Read the model definition and answer for the solid it produces. Units are mm, in the model's axes. A direction names the side the tool comes from. Coordinates: 2 decimals unless noted, no trailing zeros. Write each loop counter-clockwise with the first axis right and the second up, starting at its lowest first coordinate (ties: lowest second). Pieces come first, ordered by that corner, then holes. Notation, with made-up numbers: (87, 84) -> (98, 84) arc R29 cw to (98, 122) -> close; hole circle Ø1 at (72.5, 26). An arc over 180 degrees is marked (long way). Use CSV: the item, a comma, the result in double quotes.
from build123d import *

# Parameters (mm, degrees)
SKETCH1_W           = 4.572
SKETCH1_H           = 28.575
SKETCH2_R           = 12.1666
BOSS_EXTRUDE1_DEPTH = 20.828
CUT_EXTRUDE1_DEPTH  = 26.4
SKETCH4_W           = 25.4
SKETCH4_H           = 4.0005
HOLE1_D             = 5.1816
HOLE1_DEPTH         = 25.4


with BuildPart() as part:
    # Sketch1 → Revolve1 (revolve)
    with BuildSketch(Plane.XY):
        with Locations((-15.321066246, 14.2875)):
            Rectangle(SKETCH1_W, SKETCH1_H)
    revolve(axis=Axis((-17.607066246, 0, 0), (1, 0, 0)))

    # Sketch2 → Boss-Extrude1 (add)
    with BuildSketch(Plane(origin=(-13.035066246, 0, 0), x_dir=(0, 0, -1), z_dir=(1, 0, 0))):
        Circle(SKETCH2_R)
    extrude(amount=BOSS_EXTRUDE1_DEPTH)

    # Sketch3 → Cut-Extrude1 (cut, through all)
    with BuildSketch(Plane.ZY.offset(17.607066246)):
        with BuildLine():
            Line((1.0033, 3.872646299), (1.0033, 5.0038))
            Line((1.0033, 5.0038), (-1.0033, 5.0038))
            Line((-1.0033, 5.0038), (-1.0033, 3.872646299))
            ThreePointArc((-1.0033, 3.872646299), (0, 4.0005), (1.0033, 3.872646299))
        make_face()
    extrude(amount=-CUT_EXTRUDE1_DEPTH, mode=Mode.SUBTRACT)

    # Sketch4 → Cut-Revolve1 (revolve, cut)
    with BuildSketch(Plane(origin=(0, 0, 0), x_dir=(-1, 0, 0), z_dir=(0, 0, -1))):
        with Locations((4.907066246, 2.00025)):
            Rectangle(SKETCH4_W, SKETCH4_H)
    revolve(axis=Axis((7.792933754, 0, 0), (-1, 0, 0)), mode=Mode.SUBTRACT)

    # Hole1
    with Locations(Plane.ZY.offset(17.607066246)):
        with Locations((23.8125, 0), (11.90625, 20.622229928), (-11.90625, 20.622229928), (-23.8125, 0), (-11.90625, -20.622229928), (11.90625, -20.622229928)):
            Hole(HOLE1_D / 2, depth=HOLE1_DEPTH)


solid = part.part
1. A tool of negligible diameter and unlimited length cuts with its end or side. For faces 1 (the cylindrical face through (-3, 12, 2)), 2 (the flat face through (-17.607, 0, -6)), 3 (the flat face through (-5, 5.004, 0)), from which of +Z, -Z, +X, -X, +Y, -Y can it reach the whole face along a straight path? Write none if from no direction.
Solutions:
face 1,"+X"
face 2,"+Z, -Z, -X, +Y, -Y"
face 3,"+X, -X"
2. A cutting plane is placed at D-D (z = -10). Give the vertices of the cut face in (x, y), and give its area (3 significant figures).
Solutions:
outline,"(-17.61, -26.77) -> (-13.04, -26.77) -> (-13.04, -22.38) -> (-17.61, -22.38) -> close; (-17.61, -18.87) -> (-13.04, -18.87) -> (-13.04, -6.93) -> (7.79, -6.93) -> (7.79, 6.93) -> (-13.04, 6.93) -> (-13.04, 18.87) -> (-17.61, 18.87) -> close; (-17.61, 22.38) -> (-13.04, 22.38) -> (-13.04, 26.77) -> (-17.61, 26.77) -> close"
area,"501 mm^2"
3. A cutting plane is placed at B-B (y = 0). Give the vertices of the cut face in (x, z) (1 decimal), and give its area (3 significant figures).
Solutions:
outline,"(-17.6, -28.6) -> (-13, -28.6) -> (-13, -26.4) -> (-17.6, -26.4) -> close; (-17.6, -21.2) -> (-13, -21.2) -> (-13, -12.2) -> (7.8, -12.2) -> (7.8, -4) -> (-17.6, -4) -> close; (-17.6, 4) -> (7.8, 4) -> (7.8, 12.2) -> (-13, 12.2) -> (-13, 21.2) -> (-17.6, 21.2) -> close; (-17.6, 26.4) -> (-13, 26.4) -> (-13, 28.6) -> (-17.6, 28.6) -> close"
area,"517 mm^2"
4. Each of these flat-tipped pins is pushed along its axis until it touches: pin 1 Ø6.5 at (y, z) = (-20.62, -11.91) entering from +X; pin 2 Ø12 at (x, z) = (-9.5, 5.5) entering from -Y; pin 3 Ø4 at (y, z) = (0, 23.81) entering from +X; pin 4 Ø0.6 at (x, y) = (-3, 4.5) entering from -Z. Where does it stop, or does it pass through?
Solutions:
pin 1,"stops at x = -13.04"
pin 2,"stops at y = -28.57"
pin 3,"passes through"
pin 4,"stops at z = -11.42"
5. Find the intervals of material crossed by line 1 along Y through (x, z) = (-14, 12); line 2 along Y through (x, z) = (-13.25, 13.5); line 3 along Y through (x, z) = (2, 0), in increasing order.
Solutions:
line 1,"y = -25.93 to -23.21, -18.03 to 18.03, 23.21 to 25.93"
line 2,"y = -25.18 to -22.66, -18.58 to 18.58, 22.66 to 25.18"
line 3,"y = -12.17 to -4, 5 to 12.17"
6. A cutting plane is placed at A-A (z = 0). Give the vertices of the cut face in (x, y) (1 decimal), and give its area (3 significant figures).
Solutions:
outline,"(-17.6, -28.6) -> (-13, -28.6) -> (-13, -12.2) -> (7.8, -12.2) -> (7.8, -4) -> (-17.6, -4) -> close; (-17.6, 5) -> (7.8, 5) -> (7.8, 12.2) -> (-13, 12.2) -> (-13, 28.6) -> (-17.6, 28.6) -> close"
area,"539 mm^2"
7. For a pull along Z with two mould halves and no side action, classify faces 4 (the cylindrical face through (-15.289, -28.547, 1.256)), 5 (the cylindrical face through (-15.289, 0.778, -26.284)), 6 (the flat face through (-13.035, -12, -6)) as pulls with the +Z half, pulls with the -Z half, needs draft (parallel to the pull), parting line crosses it, or undercut.
Solutions:
face 4,"parting line crosses it"
face 5,"undercut"
face 6,"needs draft"
8. A cutting plane is placed at C-C (x = -4.25). Give the vertices of the cut face in (y, z), and give its area (3 significant figures).
Solutions:
outline,"circle Ø24.33 at (0, 0); hole (3.87, -1) -> (5, -1) -> (5, 1) -> (3.87, 1) arc R4 ccw (long way) to start"
area,"413 mm^2"
